Read the model definition and answer for the solid it produces. Units are mm, in the model's axes. A direction names the side the tool comes from. Coordinates: 2 decimals unless noted, no trailing zeros. Order: outer loops, then holes, each group sorted by start corner. A loop starts at its lowest first (then second) coordinate and runs counter-clockwise, first axis right, second up. Notation, with made-up numbers: (36.5, 33.25) -> (45.5, 33.25) arc R22 ccw to (45.5, 53.25) -> close; hole circle Ø7 at (75.25, 76.25). An arc over 180 degrees is marked (long way). Answer as a JSON object with one key per item and string values. Group by question number.
1) A tool of negligible diameter and unlimited length cuts with its end or side. For faces 1 (the flat face through (8, 9, -28)), 2 (the cylindrical face through (-9.146, 6.972, -29.609)), from which of +Z, -Z, +X, -X, +Y, -Y can it reach the whole face along a straight path? Write none if from no direction.
2) Section A-A on z = -27.5 is taken. Determine the outline of the cut face in (x, y), and give its area (3 significant figures).
3) Section C-C on z = 0 is taken. Determine the outline of the cut face in (x, y), and give its area (3 significant figures).
4) Section B-B on x = 17 is taken. Determine the outline of the cut face in (y, z).
5) Given pin 1 (12 mm diameter, centred on x = 15.5, z = -55, fed in from +Y), flat-ended and moving along its own axis, determine where the tip first touches the part or whether it passes through.
6) Determine the mould class of faces 3 (the cylindrical face through (30.248, 2.535, 74.287)), 4 (the cylindrical face through (-8.583, 6.972, -40.566)), 5 (the flat face through (0, 2, 75)), 6 (the flat face through (-31, 2, 1)) for opening direction X: released by +X, released by -X, zero draft, split by the parting line, or undercut.
7) Consider L1, parallel to Z at x = -8, y = 6; L2, parallel to Y at x = -15.5, z = 27.5. Determine where each line is inside the solid, lowest interval first.
from build123d import *

# Parameters (mm, degrees)
SKETCH1_W           = 62
SKETCH1_H           = 150
BOSS_EXTRUDE1_DEPTH = 5
FILLET1_R           = 2.5
SKETCH3_R           = 2.5
BOSS_EXTRUDE2_DEPTH = 4


with BuildPart() as part:
    # Sketch1 → Boss-Extrude1 (new body)
    with BuildSketch(Plane(origin=(0, 0, 0), x_dir=(1, 0, 0), z_dir=(0, 1, 0))):
        Rectangle(SKETCH1_W, SKETCH1_H)
    extrude(amount=BOSS_EXTRUDE1_DEPTH)

    # Fillet1
    fillet1_edges = [part.edges().sort_by_distance(p)[0] for p in [
        (31, 2.5, 75),
        (-31, 2.5, 75),
        (-31, 2.5, -75),
        (31, 2.5, -75),
    ]]
    fillet(fillet1_edges, radius=FILLET1_R)

    # Sketch3 → Boss-Extrude2 (add)
    with BuildSketch(Plane(origin=(0, 5, 0), x_dir=(1, 0, 0), z_dir=(0, 1, 0))):
        with Locations(Location((-7.625, 42.875, 0), (0, 0, 270))):
            Circle(SKETCH3_R)
        with Locations(Location((7.625, 42.875, 0), (0, 0, 270))):
            Circle(SKETCH3_R)
        with Locations(Location((7.625, 27.625, 0), (0, 0, 270))):
            Circle(SKETCH3_R)
        with Locations(Location((-7.625, 27.625, 0), (0, 0, 270))):
            Circle(SKETCH3_R)
    extrude(amount=BOSS_EXTRUDE2_DEPTH)


solid = part.part
Worked answers:
{
 "1": {"face 1": "+Z, -Z, +X, -X, +Y", "face 2": "+Y"},
 "2": {"outline": "(-31, 0) -> (31, 0) -> (31, 5) -> (10.12, 5) -> (10.12, 9) -> (5.13, 9) -> (5.13, 5) -> (-5.13, 5) -> (-5.13, 9) -> (-10.12, 9) -> (-10.12, 5) -> (-31, 5) -> close", "area": "350 mm²"},
 "3": {"outline": "(-31, 0) -> (31, 0) -> (31, 5) -> (-31, 5) -> close", "area": "310 mm²"},
 "4": {"outline": "(0, -75) -> (5, -75) -> (5, 75) -> (0, 75) -> close"},
 "5": {"pin 1": "stops at y = 5"},
 "6": {"face 3": "released by +X", "face 4": "undercut", "face 5": "zero draft", "face 6": "released by -X"},
 "7": {"L1": "z = -45.35 to -40.4, -30.1 to -25.15", "L2": "y = 0 to 5"}
}
